Model file for the job. Use its own axes, mm. A direction names the side the tool comes from. Round coordinates to 2 decimals unless told otherwise and drop trailing zeros. Loops run counter-clockwise (first coordinate to the right, second up) from the corner with the lowest first, then second, coordinate; pieces in that order, holes last. Notation, with made-up numbers: M -9,-25 L 22,-25 A10 ccw 22,-14 Z; hole C 62,-33.5 d10. An arc over 180 degrees is marked long. Use a Markdown table: item, result. Add a question column.
Q1. Mould opens along Z. For faces 1 (the face through (11.82, 14.43, 1.03)), 2 (the face through (18, 10, -7.5)), 3 (the face through (-1.187, 13.098, -1.547)) say: +Z half, -Z half, draft (parallel to the pull), parting line (faces both ways), or undercut.
Q2. Cut at A-A (x = 9). Give the cut face in (y, z), plus the area to 3 significant figures.
Q3. Cut at D-D (x = 18.25). Give the cut face in (y, z).
Q4. Cut at B-B (y = 10). State how many separate pieces and enclosed holes the cut face has, plus the area to 3 significant figures.
Q5. Probe line 1 (Y direction, x = 16, z = -21.5); line 2 (X direction, y = 13.5, z = -6); line 3 (Y direction, x = 18.25, z = 10.5). List the from-to ranges inside material, lowest first. Write a range as from..to.
Q6. Pin check, flat tips, straight feed: pin 1 (2.5 mm diameter, centred on x = -0.25, y = 10, fed in from +Z); pin 2 (6.5 mm diameter, centred on x = 0, z = 0, fed in from +Y); pin 3 (2 mm diameter, centred on x = -19, y = 21.5, fed in from +Z). Stop position of each tip, or through.
Q7. Tool access for faces 4 (the face through (19.589, 9.445, -13.204)), 5 (the face through (-20, 20, 2)), 6 (the face through (19.589, 9.445, 13.964)), 7 (the face through (15, 21, 2)): list every direction of +Z, -Z, +X, -X, +Y, -Y with a clear straight run to the whole face (end or side of a thin tool).
from build123d import *

# Parameters (mm, degrees)
SKICA4_W                  = 50
SKICA4_H                  = 50
P_IDAT_VYSUNUT_M2_DEPTH   = 20
ODEBRAT_VYSUNUT_M3_DEPTH  = 3.5
SKICA6_R                  = 1.45
ODEBRAT_VYSUNUT_M4_DEPTH  = 14
SKICA7_R                  = 5.25
ODEBRAT_VYSUNUT_M5_DEPTH  = 57.455734873
SKICA8_R                  = 7.55
ODEBRAT_VYSUNUT_M6_DEPTH  = 60.371710435
P_IDAT_VYSUNUT_M4_DEPTH   = 50
SKICA12_R                 = 1.95
ODEBRAT_VYSUNUT_M7_DEPTH  = 41.620192023
SKICA13_R                 = 4
ODEBRAT_VYSUNUT_M8_DEPTH  = 6
P_IDAT_VYSUNUT_M5_REACH   = 63.938
SKICA14_W                 = 3.7
SKICA14_H                 = 6.67
ZKOSEN_1_SIZE             = 1
ODEBRAT_VYSUNUT_M9_DEPTH  = 2
ODEBRAT_VYSUNUT_M10_DEPTH = 0.5
ZKOSEN_2_SIZE             = 0.75
ZKOSEN_3_SIZE             = 4


with BuildPart() as part:
    # Skica4 → Přidat vysunutím2 (new body)
    with BuildSketch(Plane(origin=(0, 0, 0), x_dir=(1, 0, 0), z_dir=(0, 1, 0))):
        Rectangle(SKICA4_W, SKICA4_H)
    extrude(amount=P_IDAT_VYSUNUT_M2_DEPTH)

    # Skica5 → Odebrat vysunutím3 (cut)
    with BuildSketch(Plane.XY.offset(25)):
        with BuildLine():
            Line((-1.677078252, 16.5), (19.677078252, 16.5))
            ThreePointArc((19.677078252, 16.5), (21.5, 10), (19.677078252, 3.5))
            Line((19.677078252, 3.5), (-1.677078252, 3.5))
            ThreePointArc((-1.677078252, 3.5), (-3.5, 10), (-1.677078252, 16.5))
        make_face()
    odebrat_vysunut_m3 = extrude(amount=-ODEBRAT_VYSUNUT_M3_DEPTH, mode=Mode.SUBTRACT)

    # Skica6 → Odebrat vysunutím4 (cut)
    with BuildSketch(Plane.XY.offset(21.5)):
        with Locations((-0.25, 10)):
            Circle(SKICA6_R)
        with Locations((18.25, 10)):
            Circle(SKICA6_R)
    odebrat_vysunut_m4 = extrude(amount=-ODEBRAT_VYSUNUT_M4_DEPTH, mode=Mode.SUBTRACT)

    # Zrcadlit1: Odebrat vysunutím3, Odebrat vysunutím4 across plane
    add(odebrat_vysunut_m3.mirror(Plane.XY), mode=Mode.SUBTRACT)
    add(odebrat_vysunut_m4.mirror(Plane.XY), mode=Mode.SUBTRACT)

    # Skica7 → Odebrat vysunutím5 (cut, through all)
    with BuildSketch(Plane.XY.offset(21.5)):
        with Locations((9, 10)):
            Circle(SKICA7_R)
    extrude(amount=-ODEBRAT_VYSUNUT_M5_DEPTH, mode=Mode.SUBTRACT)

    # Skica8 → Odebrat vysunutím6 (cut, through all)
    with BuildSketch(Plane.XY.offset(25)):
        with Locations((-15, 10)):
            Circle(SKICA8_R)
    extrude(amount=-ODEBRAT_VYSUNUT_M6_DEPTH, mode=Mode.SUBTRACT)

    # Skica11 → Přidat vysunutím4 (add)
    with BuildSketch(Plane(origin=(0, 0, -25), x_dir=(-1, 0, 0), z_dir=(0, 0, -1))):
        Polygon((-15, 20), (-15, 22.67), (-13.833651513, 24.06), (-13.833651513, 24.61), (-15, 26), (-15, 26.47), (-14.8, 26.67), (-5.2, 26.67), (-5, 26.47), (-5, 26), (-6.166348487, 24.61), (-6.166348487, 24.06), (-5, 22.67), (-5, 20), align=None)
        Polygon((15, 20), (15, 22.67), (13.833651513, 24.06), (13.833651513, 24.61), (15, 26), (15, 26.47), (14.8, 26.67), (5.2, 26.67), (5, 26.47), (5, 26), (6.166348487, 24.61), (6.166348487, 24.06), (5, 22.67), (5, 20), align=None)
    extrude(amount=-P_IDAT_VYSUNUT_M4_DEPTH)

    # Skica12 → Odebrat vysunutím7 (cut, through all)
    with BuildSketch(Plane(origin=(0, 20, 0), x_dir=(1, 0, 0), z_dir=(0, 1, 0))):
        with Locations(Location((0, 0, 0), (0, 0, 270))):
            Circle(SKICA12_R)
    extrude(amount=-ODEBRAT_VYSUNUT_M7_DEPTH, mode=Mode.SUBTRACT)

    # Skica13 → Odebrat vysunutím8 (cut)
    with BuildSketch(Plane.XZ):
        with Locations(Location((0, 0, 0), (0, 0, 270))):
            Circle(SKICA13_R)
    extrude(amount=-ODEBRAT_VYSUNUT_M8_DEPTH, mode=Mode.SUBTRACT)

    # Přidat vysunutím5: up to this face of the body (flat: up to its plane)
    p_idat_vysunut_m5_end = Plane(part.part.faces().sort_by_distance((-25, 10, 0))[0])
    # Skica14 → Přidat vysunutím5 (add, up to the picked face)
    with BuildSketch(Plane(origin=(25, 0, 0), x_dir=(0, 0, -1), z_dir=(1, 0, 0)), mode=Mode.PRIVATE) as p_idat_vysunut_m5_sk1:
        with Locations((23.15, 23.335)):
            Rectangle(SKICA14_W, SKICA14_H)
    p_idat_vysunut_m5_tool1 = split(extrude(p_idat_vysunut_m5_sk1.sketch, amount=-P_IDAT_VYSUNUT_M5_REACH, mode=Mode.PRIVATE), bisect_by=p_idat_vysunut_m5_end, keep=Keep.BOTH, mode=Mode.PRIVATE)
    add(p_idat_vysunut_m5_tool1.solids().sort_by(Axis((25, 23.335, -23.15), (-1, 0, 0)))[0])

    # Zkosení1
    zkosen_1_edges = [part.edges().sort_by_distance(p)[0] for p in [
        (-22.55, 10, 25),
    ]]
    chamfer(zkosen_1_edges, length=ZKOSEN_1_SIZE)

    # Skica16 → Odebrat vysunutím9 (cut)
    with BuildSketch(Plane(origin=(0, 0, -21.5), x_dir=(-1, 0, 0), z_dir=(0, 0, -1))):
        with BuildLine():
            Line((1.677078252, 16.5), (-19.677078252, 16.5))
            ThreePointArc((-19.677078252, 16.5), (-21.5, 10), (-19.677078252, 3.5))
            Line((-19.677078252, 3.5), (1.677078252, 3.5))
            ThreePointArc((1.677078252, 3.5), (3.5, 10), (1.677078252, 16.5))
        make_face()
    extrude(amount=-ODEBRAT_VYSUNUT_M9_DEPTH, mode=Mode.SUBTRACT)

    # Skica17 → Odebrat vysunutím10 (cut)
    with BuildSketch(Plane.XY.offset(21.5)):
        with BuildLine():
            Line((-1.677078252, 3.5), (19.677078252, 3.5))
            ThreePointArc((19.677078252, 3.5), (21.5, 10), (19.677078252, 16.5))
            Line((19.677078252, 16.5), (-1.677078252, 16.5))
            ThreePointArc((-1.677078252, 16.5), (-3.5, 10), (-1.677078252, 3.5))
        make_face()
    extrude(amount=-ODEBRAT_VYSUNUT_M10_DEPTH, mode=Mode.SUBTRACT)

    # Zkosení2
    zkosen_2_edges = [part.edges().sort_by_distance(p)[0] for p in [
        (16.8, 10, -19.5),
        (-1.7, 10, -19.5),
        (16.8, 10, 21),
        (-1.7, 10, 21),
    ]]
    chamfer(zkosen_2_edges, length=ZKOSEN_2_SIZE)

    # Zkosení3
    zkosen_3_edges = [part.edges().sort_by_distance(p)[0] for p in [
        (25, 26.67, -23.15),
        (-25, 26.67, -23.15),
    ]]
    chamfer(zkosen_3_edges, length=ZKOSEN_3_SIZE)


solid = part.part
Checked values:
| question | item | result |
|---|---|---|
| 1 | face 1 | draft |
| 1 | face 2 | -Z half |
| 1 | face 3 | undercut |
| 2 | outline | M 0,-25 L 3.5,-25 L 3.5,-19.5 L 4.75,-19.5 L 4.75,21 L 3.5,21 L 3.5,25 L 0,25 Z; M 15.25,-19.5 L 16.5,-19.5 L 16.5,-25 L 26.67,-25 L 26.67,25 L 16.5,25 L 16.5,21 L 15.25,21 Z |
| 2 | area | 785 mm^2 |
| 3 | outline | M 0,-25 L 3.5,-25 L 3.5,-19.5 L 7.8,-19.5 L 8.55,-18.75 L 8.55,-7.5 L 11.45,-7.5 L 11.45,-18.75 L 12.2,-19.5 L 16.5,-19.5 L 16.5,-25 L 26.67,-25 L 26.67,-21.3 L 20,-21.3 L 20,25 L 16.5,25 L 16.5,21 L 12.2,21 L 11.45,20.25 L 11.45,7.5 L 8.55,7.5 L 8.55,20.25 L 7.8,21 L 3.5,21 L 3.5,25 L 0,25 Z |
| 4 | separate pieces | 3 |
| 4 | enclosed holes | 1 |
| 4 | area | 919 mm^2 |
| 5 | line 1 | y = 0..3.5, 16.5..26.67 |
| 5 | line 2 | x = -25..-21.69, -8.31..5.09, 12.91..25 |
| 5 | line 3 | y = 0..8.55, 11.45..20 |
| 6 | pin 1 | stops at z = 7.5 |
| 6 | pin 2 | stops at y = 20 |
| 6 | pin 3 | stops at z = -21.3 |
| 7 | face 4 | -Z |
| 7 | face 5 | +Z, -X, +Y |
| 7 | face 6 | +Z |
| 7 | face 7 | +Z, +X, +Y |
